For this review, use the dimensioned drawing (mm, ordinates from the lowest corner) and the shaded views. A direction names the side the tool comes from. Give positions to 0.01 mm unless a question says otherwise; leave off trailing zeros. Order: outer loops, then holes, each group sorted by start corner. A loop starts at its lowest first (then second) coordinate and runs counter-clockwise, first axis right, second up. Notation, with made-up numbers: (70.5, -3) - (84.5, -3) arc R29 ccw to (84.5, 32) - close; hole circle Ø11 at (37, -21.5). An arc over 180 degrees is marked (long way). Use a Markdown table: item, result. Add a question column.
1) Wall thickness on L1, parallel to X at y = 24.05, z = 26.15 (1 decimal); L2, parallel to Y at x = 32, z = 11; L3, parallel to Y at x = 26.5, z = 32: over which ranges is each line inside the solid? List them lowest first.
2) Machinability: for the marked faces 1, 2 and 3, which of the approach directions +Z, -Z, +X, -X, +Y, -Y give a long, thin tool a straight path to every point of the face, cutting with its end or side? Answer none if there is none.
3) Clearance check with flat-ended pins moving along their axes: P1, Ø2, axis at x = 7, z = 13.5, coming from the -Y side; P2, Ø12, axis at x = 16.5, y = 42, coming from the -Z side; P3, Ø1, axis at y = 24.5, z = 22, coming from the -X side. State where each tip first meets the part, or that it passes through.
4) We need section C-C on y = 68.5. Write out the cut boundary in (x, z).
5) We need section B-B on y = 26. Write out the cut boundary in (x, z).
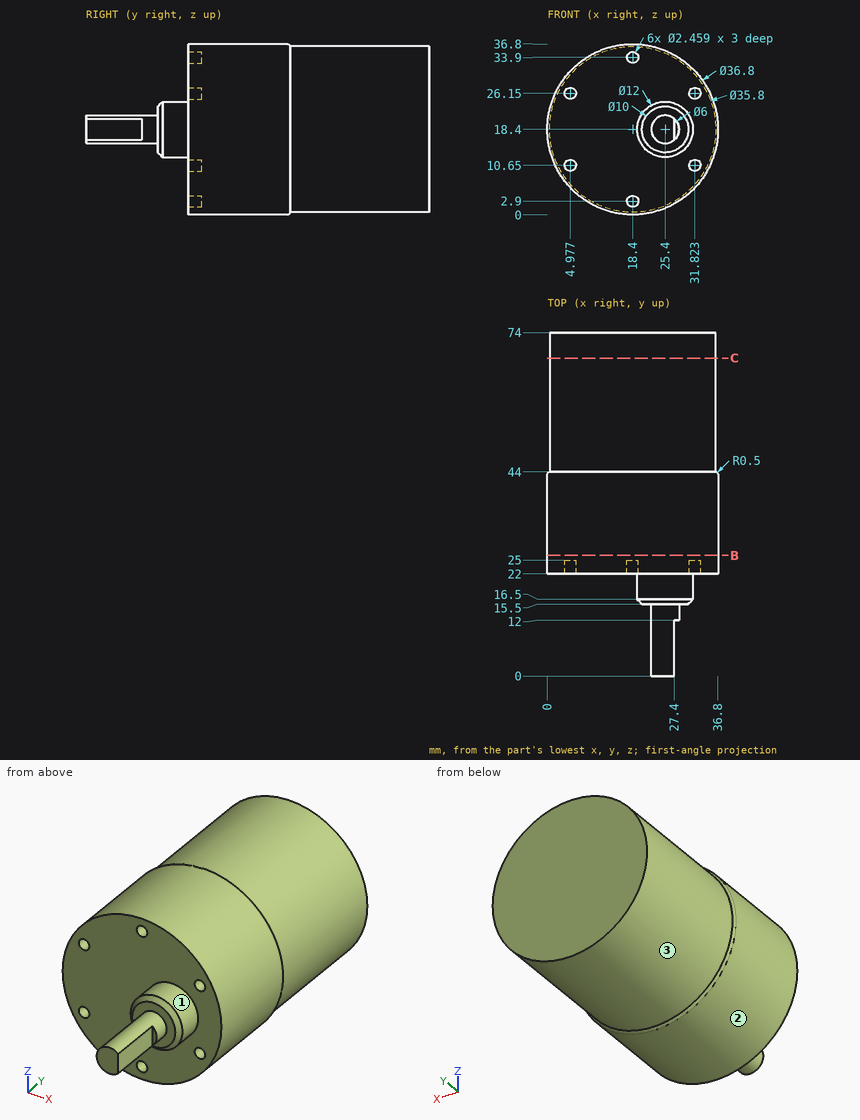
Checked values:
| question | item | result |
|---|---|---|
| 1 | L1 | 1.7 to 3.7, 6.2 to 30.6, 33.1 to 35.1 |
| 1 | L2 | 25 to 74 |
| 1 | L3 | 22 to 74 |
| 2 | face 1 | -Y |
| 2 | face 2 | +Y, -Y |
| 2 | face 3 | +Y |
| 3 | P1 | y = 22 |
| 3 | P2 | z = 0 |
| 3 | P3 | x = 0.26 |
| 4 | outline | circle Ø35.8 at (18.4, 18.4) |
| 5 | outline | circle Ø36.8 at (18.4, 18.4) |
